For this review, take the finished solid that the model builds, in its own axes (mm). Face numbers are marked on the shaded views. A direction names the side the tool comes from. Round coordinates to 2 decimals unless told otherwise and drop trailing zeros. Write each loop counter-clockwise with the first axis right and the second up, starting at its lowest first coordinate (ties: lowest second). Pieces come first, ordered by that corner, then holes. Notation, with made-up numbers: (-11.5, -18) -> (5.5, -18) arc R22 cw to (5.5, 11) -> close; hole circle Ø8 at (80.25, 45.25). An arc over 180 degrees is marked (long way). Answer in a Markdown table with one row per item.
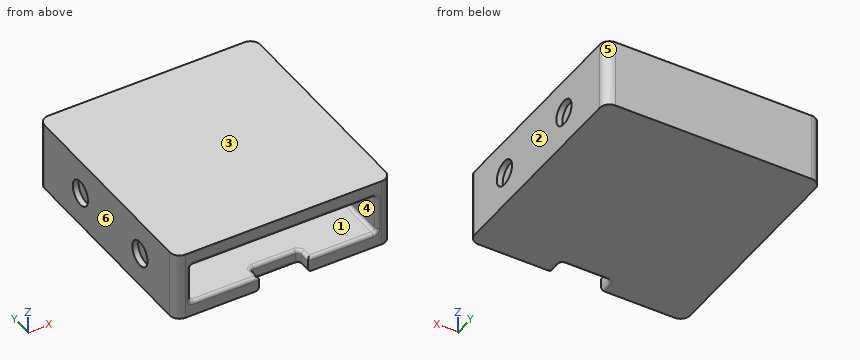
from build123d import *

# Parameters (mm, degrees)
BOSS_EXTRUDE4_DEPTH = 3
BOSS_EXTRUDE5_DEPTH = 14
BOSS_EXTRUDE6_START = 11
BOSS_EXTRUDE6_DEPTH = 3
SKETCH2_W           = 10
SKETCH2_H           = 3
CUT_EXTRUDE1_DEPTH  = 3
CUT_EXTRUDE2_START  = 22
SKETCH3_R           = 2.55
CUT_EXTRUDE2_DEPTH  = 1.2
CUT_EXTRUDE3_START  = -20.8
SKETCH3_3_R         = 2.55
CUT_EXTRUDE3_DEPTH  = 1.2
FILLET1_R           = 0.7


with BuildPart() as part:
    # Sketch1 → Boss-Extrude4 (new body)
    with BuildSketch(Plane.XY.offset(31)):
        with BuildLine():
            ThreePointArc((-22, -20), (-21.414213562, -21.414213562), (-20, -22))
            Line((-20, -22), (20, -22))
            ThreePointArc((20, -22), (21.414213562, -21.414213562), (22, -20))
            Line((22, -20), (22, 22))
            ThreePointArc((22, 22), (21.414213562, 23.414213562), (20, 24))
            Line((20, 24), (-20, 24))
            ThreePointArc((-20, 24), (-21.414213562, 23.414213562), (-22, 22))
            Line((-22, 22), (-22, -20))
        make_face()
    extrude(amount=BOSS_EXTRUDE4_DEPTH)

    # Sketch1<3> → Boss-Extrude5 (add)
    with BuildSketch(Plane.XY.offset(31)):
        with BuildLine():
            Line((-22, -10.75), (-22, -20))
            ThreePointArc((-22, -20), (-21.414213562, -21.414213562), (-20, -22))
            Line((-20, -22), (-19, -22))
            Line((-19, -22), (-19, -18))
            Line((-19, -18), (-19, -10.75))
            Line((-19, -10.75), (-19, 10.75))
            Line((-19, 10.75), (-19, 20))
            ThreePointArc((-19, 20), (-18.707106781, 20.707106781), (-18, 21))
            Line((-18, 21), (-3.938916155, 21))
            Line((-3.938916155, 21), (3.938916155, 21))
            Line((3.938916155, 21), (18, 21))
            ThreePointArc((18, 21), (18.707106781, 20.707106781), (19, 20))
            Line((19, 20), (19, 10.75))
            Line((19, 10.75), (19, -10.75))
            Line((19, -10.75), (19, -18))
            Line((19, -18), (19, -22))
            Line((19, -22), (20, -22))
            ThreePointArc((20, -22), (21.414213562, -21.414213562), (22, -20))
            Line((22, -20), (22, -10.75))
            Line((22, -10.75), (22, 10.75))
            Line((22, 10.75), (22, 22))
            ThreePointArc((22, 22), (21.414213562, 23.414213562), (20, 24))
            Line((20, 24), (3.938916155, 24))
            Line((3.938916155, 24), (-3.938916155, 24))
            Line((-3.938916155, 24), (-20, 24))
            ThreePointArc((-20, 24), (-21.414213562, 23.414213562), (-22, 22))
            Line((-22, 22), (-22, 10.75))
            Line((-22, 10.75), (-22, -10.75))
        make_face()
    extrude(amount=BOSS_EXTRUDE5_DEPTH)

    # Sketch1<4> → Boss-Extrude6 (add)
    # profile 1 of 3: a face of its own
    with BuildSketch(Plane.XY.offset(31).offset(BOSS_EXTRUDE6_START)):
        with BuildLine():
            Line((-22, -20), (-22, -10.75))
            Line((-22, -10.75), (-22, 10.75))
            Line((-22, 10.75), (-22, 22))
            ThreePointArc((-22, 22), (-21.414213562, 23.414213562), (-20, 24))
            Line((-20, 24), (-3.938916155, 24))
            Line((-3.938916155, 24), (3.938916155, 24))
            Line((3.938916155, 24), (20, 24))
            ThreePointArc((20, 24), (21.414213562, 23.414213562), (22, 22))
            Line((22, 22), (22, 10.75))
            Line((22, 10.75), (22, -10.75))
            Line((22, -10.75), (22, -20))
            ThreePointArc((22, -20), (21.414213562, -21.414213562), (20, -22))
            Line((20, -22), (10.75, -22))
            Line((10.75, -22), (-10.75, -22))
            Line((-10.75, -22), (-20, -22))
            ThreePointArc((-20, -22), (-21.414213562, -21.414213562), (-22, -20))
        make_face()
        with BuildLine():
            ThreePointArc((-18, 21), (-18.707106781, 20.707106781), (-19, 20))
            Line((-19, 20), (-19, 10.75))
            Line((-19, 10.75), (-19, -10.75))
            Line((-19, -10.75), (-19, -18))
            ThreePointArc((-19, -18), (-18.707106781, -18.707106781), (-18, -19))
            Line((-18, -19), (-10.75, -19))
            Line((-10.75, -19), (10.75, -19))
            Line((10.75, -19), (18, -19))
            ThreePointArc((18, -19), (18.707106781, -18.707106781), (19, -18))
            Line((19, -18), (19, -10.75))
            Line((19, -10.75), (19, 10.75))
            Line((19, 10.75), (19, 20))
            ThreePointArc((19, 20), (18.707106781, 20.707106781), (18, 21))
            Line((18, 21), (3.938916155, 21))
            Line((3.938916155, 21), (-3.938916155, 21))
            Line((-3.938916155, 21), (-18, 21))
        make_face(mode=Mode.SUBTRACT)
    # profile 2 of 3: a face of its own
    with BuildSketch(Plane.XY.offset(31).offset(BOSS_EXTRUDE6_START)):
        with BuildLine():
            Line((-18, 21), (-3.938916155, 21))
            Line((-3.938916155, 21), (3.938916155, 21))
            Line((3.938916155, 21), (18, 21))
            ThreePointArc((18, 21), (18.707106781, 20.707106781), (19, 20))
            Line((19, 20), (19, 10.75))
            Line((19, 10.75), (19, -10.75))
            Line((19, -10.75), (19, -18))
            ThreePointArc((19, -18), (18.707106781, -18.707106781), (18, -19))
            Line((18, -19), (10.75, -19))
            Line((10.75, -19), (-10.75, -19))
            Line((-10.75, -19), (-18, -19))
            ThreePointArc((-18, -19), (-18.707106781, -18.707106781), (-19, -18))
            Line((-19, -18), (-19, -10.75))
            Line((-19, -10.75), (-19, 10.75))
            Line((-19, 10.75), (-19, 20))
            ThreePointArc((-19, 20), (-18.707106781, 20.707106781), (-18, 21))
        make_face()
    # profile 3 of 3: a face of its own
    with BuildSketch(Plane.XY.offset(31).offset(BOSS_EXTRUDE6_START)):
        with BuildLine():
            Line((-19, -18), (-19, -22))
            Line((-19, -22), (-10.75, -22))
            Line((-10.75, -22), (10.75, -22))
            Line((10.75, -22), (19, -22))
            Line((19, -22), (19, -18))
            ThreePointArc((19, -18), (18.707106781, -18.707106781), (18, -19))
            Line((18, -19), (10.75, -19))
            Line((10.75, -19), (-10.75, -19))
            Line((-10.75, -19), (-18, -19))
            ThreePointArc((-18, -19), (-18.707106781, -18.707106781), (-19, -18))
        make_face()
    extrude(amount=BOSS_EXTRUDE6_DEPTH)

    # Sketch2 → Cut-Extrude1 (cut)
    with BuildSketch(Plane.XZ.offset(22)):
        with Locations((0, 32.5)):
            Rectangle(SKETCH2_W, SKETCH2_H)
        with Locations((0, 35.5)):
            Rectangle(SKETCH2_W, SKETCH2_H)
    extrude(amount=-CUT_EXTRUDE1_DEPTH, mode=Mode.SUBTRACT)

    # Sketch3 → Cut-Extrude2 (cut)
    with BuildSketch(Plane(origin=(0, 0, 0), x_dir=(0, 0, -1), z_dir=(1, 0, 0)).offset(CUT_EXTRUDE2_START)):
        with Locations(Location((-38, 10, 0), (0, 0, 90))):
            Circle(SKETCH3_R)
        with Locations(Location((-38, -10, 0), (0, 0, 90))):
            Circle(SKETCH3_R)
    extrude(amount=-CUT_EXTRUDE2_DEPTH, mode=Mode.SUBTRACT)

    # Sketch3<3> → Cut-Extrude3 (cut)
    with BuildSketch(Plane(origin=(0, 0, 0), x_dir=(0, 0, -1), z_dir=(1, 0, 0)).offset(CUT_EXTRUDE3_START)):
        with Locations(Location((-38, -10, 0), (0, 0, 90))):
            Circle(SKETCH3_3_R)
        with Locations(Location((-38, 10, 0), (0, 0, 90))):
            Circle(SKETCH3_3_R)
    extrude(amount=-CUT_EXTRUDE3_DEPTH, mode=Mode.SUBTRACT)

    # Fillet1
    fillet1_edges = [part.edges().sort_by_distance(p)[0] for p in [
        (-19, -22, 38),
        (0, -22, 42),
        (0, 21, 42),
        (19, -1, 42),
        (-19, -1, 42),
        (18.707106781, 20.707106781, 42),
        (-12, -22, 34),
        (-5, -20.5, 34),
        (5, -20.5, 34),
        (0, -19, 31),
        (5, -20.5, 31),
        (-5, -19, 32.5),
        (-5, -20.5, 31),
        (5, -19, 32.5),
        (0, -19, 34),
        (12, -22, 34),
        (19, -1, 34),
        (0, 21, 34),
        (-19, -1, 34),
        (18.707106781, 20.707106781, 34),
        (-18.707106781, 20.707106781, 34),
        (-18.707106781, 20.707106781, 42),
        (19, -22, 38),
    ]]
    fillet(fillet1_edges, radius=FILLET1_R)


solid = part.part
1) For the marked faces 1 and 2, list the 3-axis set-ups (+Z, -Z, +X, -X, +Y, -Y) from which the entire face can be reached by the end or side of a thin tool; tool diameter is ignored.
Solved:
| item | result |
|---|---|
| face 1 | -Y |
| face 2 | +Z, -Z, +X, +Y, -Y |
2) For line 1 (Z direction, x = 8, y = -19); line 2 (X direction, y = 4.5, z = 38); line 3 (X direction, y = 9, z = 38.75), list the stretches that pass through material, from the lowest coordinate up. Write a range as [from, to].
Solved:
| item | result |
|---|---|
| line 1 | [31, 34], [42, 45] |
| line 2 | [-22, -19], [19, 22] |
| line 3 | [-20.8, -19], [19, 20.8] |
3) Mouldability with a two-part tool opening along X and no side actions: class the marked faces 3, 4, 5 and 6 as pulls with the +X half, pulls with the -X half, needs draft (parallel to the pull), parting line crosses it, or undercut.
Solved:
| item | result |
|---|---|
| face 3 | needs draft |
| face 4 | undercut |
| face 5 | pulls with the +X half |
| face 6 | pulls with the -X half |
4) Consider section B-B on x = 15.5. State the section outline as (y, z) points.
Solved:
| item | result |
|---|---|
| outline | (-22, 31) -> (24, 31) -> (24, 45) -> (-22, 45) -> (-22, 42.7) arc R0.7 ccw to (-21.3, 42) -> (20.3, 42) arc R0.7 cw to (21, 41.3) -> (21, 34.7) arc R0.7 cw to (20.3, 34) -> (-21.3, 34) arc R0.7 ccw to (-22, 33.3) -> close |
5) Clearance check with flat-ended pins moving along their axes: pin 1 Ø1.3 at (x, z) = (-2, 32) entering from -Y; pin 2 Ø2 at (x, z) = (1, 40.5) entering from -Y; pin 3 Ø2.5 at (y, z) = (11, 38) entering from +X. State where each tip first meets the part, or that it passes through.
Solved:
| item | result |
|---|---|
| pin 1 | y = -19 |
| pin 2 | y = 20.97 |
| pin 3 | x = 20.8 |
6) Consider section A-A on y = 15. State the section outline as (x, z) points.
Solved:
| item | result |
|---|---|
| outline | (-22, 31) -> (22, 31) -> (22, 45) -> (-22, 45) -> close; hole (-19, 34.7) arc R0.7 ccw to (-18.3, 34) -> (18.3, 34) arc R0.7 ccw to (19, 34.7) -> (19, 41.3) arc R0.7 ccw to (18.3, 42) -> (-18.3, 42) arc R0.7 ccw to (-19, 41.3) -> close |
7) Consider section D-D on y = -10. State the section outline as (x, z) points, then the cut area to 3 significant figures.
Solved:
| item | result |
|---|---|
| outline | (-22, 31) -> (22, 31) -> (22, 35.45) -> (20.8, 35.45) -> (20.8, 40.55) -> (22, 40.55) -> (22, 45) -> (-22, 45) -> (-22, 40.55) -> (-20.8, 40.55) -> (-20.8, 35.45) -> (-22, 35.45) -> close; hole (-19, 34.7) arc R0.7 ccw to (-18.3, 34) -> (18.3, 34) arc R0.7 ccw to (19, 34.7) -> (19, 41.3) arc R0.7 ccw to (18.3, 42) -> (-18.3, 42) arc R0.7 ccw to (-19, 41.3) -> close |
| area | 300 mm² |
